Source: CAD feature listing. Evaluate the final solid. Frame: model axes, mm. Coordinates: 2 decimals unless noted, no trailing zeros.
```python
from build123d import *

# Parameters (mm, degrees)
BOSS_EXTRUDE1_DEPTH = 1.6
CUT_EXTRUDE1_DEPTH  = 0.8


with BuildPart() as part:
    # Sketch1 → Boss-Extrude1 (new body)
    with BuildSketch(Plane(origin=(0, 0, 0), x_dir=(1, 0, 0), z_dir=(0, 1, 0))):
        Polygon((0, -60), (51.961524227, -30), (51.961524227, 30), (0, 60), (-51.961524227, 30), (-51.961524227, -30), align=None)
    extrude(amount=BOSS_EXTRUDE1_DEPTH)

    # Sketch2 → Cut-Extrude1 (cut)
    # profile 1 of 4: a face of its own
    with BuildSketch(Plane(origin=(0, 1.6, 0), x_dir=(1, 0, 0), z_dir=(0, 1, 0))):
        Polygon((0, 58.845299462), (-50.961524227, 29.422649731), (-50.961524227, -29.422649731), (0, -58.845299462), (50.961524227, -29.422649731), (50.961524227, 29.422649731), align=None)
        Polygon((-49.961524227, 28.845299462), (-49.961524227, -28.845299462), (0, -57.690598923), (49.961524227, -28.845299462), (49.961524227, 28.845299462), (0, 57.690598923), align=None, mode=Mode.SUBTRACT)
    # profile 2 of 4: a face of its own
    with BuildSketch(Plane(origin=(0, 1.6, 0), x_dir=(1, 0, 0), z_dir=(0, 1, 0))):
        Polygon((0, 56.535898385), (-48.961524227, 28.267949192), (-48.961524227, -28.267949192), (0, -56.535898385), (48.961524227, -28.267949192), (48.961524227, 28.267949192), align=None)
        Polygon((-47.961524227, 27.690598923), (-47.961524227, -27.690598923), (0, -55.381197846), (47.961524227, -27.690598923), (47.961524227, 27.690598923), (0, 55.381197846), align=None, mode=Mode.SUBTRACT)
    # profile 3 of 4: a face of its own
    with BuildSketch(Plane(origin=(0, 1.6, 0), x_dir=(1, 0, 0), z_dir=(0, 1, 0))):
        Polygon((0, 54.226497308), (-46.961524227, 27.113248654), (-46.961524227, -27.113248654), (0, -54.226497308), (46.961524227, -27.113248654), (46.961524227, 27.113248654), align=None)
        Polygon((-45.961524227, 26.535898385), (-45.961524227, -26.535898385), (0, -53.07179677), (45.961524227, -26.535898385), (45.961524227, 26.535898385), (0, 53.07179677), align=None, mode=Mode.SUBTRACT)
    # profile 4 of 4: a face of its own
    with BuildSketch(Plane(origin=(0, 1.6, 0), x_dir=(1, 0, 0), z_dir=(0, 1, 0))):
        Polygon((0, 51.917096231), (-44.961524227, 25.958548116), (-44.961524227, -25.958548116), (0, -51.917096231), (44.961524227, -25.958548116), (44.961524227, 25.958548116), align=None)
        Polygon((-43.961524227, 25.381197846), (-43.961524227, -25.381197846), (0, -50.762395693), (43.961524227, -25.381197846), (43.961524227, 25.381197846), (0, 50.762395693), align=None, mode=Mode.SUBTRACT)
    extrude(amount=-CUT_EXTRUDE1_DEPTH, mode=Mode.SUBTRACT)


solid = part.part
```
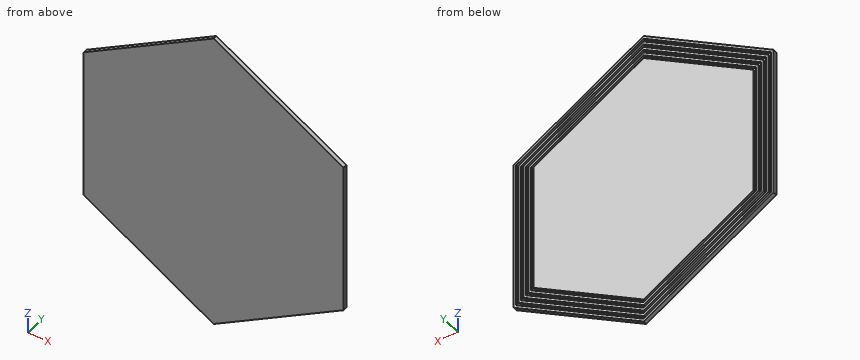
Q1. Pin query (flat end, axial travel): P1, Ø12, axis at x = -14, z = -39.5, coming from the -Y side. Return the tip coordinate at first contact, or that it passes through.
Solutions:
P1: stops at y = 0
Q2. Section query A-A on y = 1.05. Give the number of separate pieces and of enclosed holes in the cut face, plus the area to 3 significant figures.
Solutions:
separate pieces: 5
enclosed holes: 4
area: 8,040 mm2
Q3. Material intervals for line 1 along Y through (x, z) = (-24, -37); line 2 along Z through (x, y) = (6, 0.55); line 3 along Z through (x, y) = (8, 0.3), sorted ascending.
Solutions:
line 1: y = 0 to 0.8
line 2: z = -56.54 to 56.54
line 3: z = -55.38 to 55.38
